Input: part model. Units: mm. Frame: model coordinates. A direction names the side the tool comes from. Coordinates: 2 decimals unless noted, no trailing zeros. Write each loop counter-clockwise with the first axis right and the second up, starting at its lowest first coordinate (ties: lowest second). Pieces come first, ordered by that corner, then holes.
1) Pin query (flat end, axial travel): pin 1 Ø5 at (y, z) = (6, -2.5) entering from -X; pin 2 Ø2 at (y, z) = (4, -4.5) entering from +X; pin 3 Ø3 at (x, y) = (17.89, 2.5) entering from -Z. Return the tip coordinate at first contact, or that it passes through.
2) Set-up query: faces 1 (the flat face through (16, 3, -18.625)), 2 (the cylindrical face through (19.63, 0.71, -20.9)), 3 (the flat face through (-2, 7, -5)). Return all of +Z, -Z, +X, -X, +Y, -Y with unobstructed straight access to the full face (end or side cutting, diameter ignored); none if empty.
3) Section query D-D (y = 5.5). Output: boundary loops of the cut face in (x, z).
4) Draft query along X for faces 4 (the cylindrical face through (0.158, 6.467, -2.465)), 5 (the cylindrical face through (-26.9, 4.25, -12.33)), 6 (the flat face through (-1, 10, -2)). Return one class per face: pulls with the +X half, pulls with the -X half, needs draft (parallel to the pull), parting line crosses it, or undercut.
5) Section query C-C (x = -6.5). Output: boundary loops of the cut face in (y, z), then the cut area to 3 significant figures.
6) Section query B-B (z = -20.75). State how many separate pieces and enclosed holes the cut face has, then the cut area to 3 significant figures.
7) Line query: L1, parallel to X at y = 2.5, z = -21.5; L2, parallel to Y at x = -19, z = -1.75; L3, parallel to Y at x = 18, z = -3. Output: solid intervals per line, ascending.
from build123d import *

# Parameters (mm, degrees)
BOSS_EXTRUDE1_DEPTH = 5
CUT_EXTRUDE1_REACH  = 39.584
SKETCH3_R           = 1.1
FILLET1_R           = 2.5
BOSS_EXTRUDE2_DEPTH = 5
SKETCH7_R           = 1.05
CUT_EXTRUDE3_DEPTH  = 5
FILLET2_R           = 5
CUT_EXTRUDE4_REACH  = 39.584
SKETCH8_W           = 5.5
SKETCH8_H           = 14.25
CHAMFER1_SIZE       = 5
FILLET3_R           = 3


with BuildPart() as part:
    # Sketch1 → Boss-Extrude1 (new body)
    with BuildSketch(Plane(origin=(0, 0, 0), x_dir=(1, 0, 0), z_dir=(0, 1, 0))):
        Polygon((-27.613970588, 0), (20.386029412, 0), (20.386029412, 23), (-27.613970588, 25), align=None)
    extrude(amount=BOSS_EXTRUDE1_DEPTH)

    # Cut-Extrude1: up to this plane
    cut_extrude1_end = Plane(origin=(-27.613970588, 5, -25), z_dir=(-0.04163054471218136, 0, 0.999133073092352))
    # Sketch3 → Cut-Extrude1 (cut, up to the surface)
    with BuildSketch(Plane.XY, mode=Mode.PRIVATE) as cut_extrude1_sk1:
        with Locations((-25.113970588, 2.5)):
            Circle(SKETCH3_R)
    cut_extrude1_tool1 = split(extrude(cut_extrude1_sk1.sketch, amount=-CUT_EXTRUDE1_REACH, mode=Mode.PRIVATE), bisect_by=cut_extrude1_end, keep=Keep.BOTH, mode=Mode.PRIVATE)
    add(cut_extrude1_tool1.solids().sort_by_distance((-25.113971, 2.5, 0))[0], mode=Mode.SUBTRACT)
    # Sketch3 → Cut-Extrude1 (cut, up to the surface)
    with BuildSketch(Plane.XY, mode=Mode.PRIVATE) as cut_extrude1_sk2:
        with Locations((17.886029412, 2.5)):
            Circle(SKETCH3_R)
    cut_extrude1_tool2 = split(extrude(cut_extrude1_sk2.sketch, amount=-CUT_EXTRUDE1_REACH, mode=Mode.PRIVATE), bisect_by=cut_extrude1_end, keep=Keep.BOTH, mode=Mode.PRIVATE)
    add(cut_extrude1_tool2.solids().sort_by_distance((17.886029, 2.5, 0))[0], mode=Mode.SUBTRACT)

    # Fillet1
    fillet1_edges = [part.edges().sort_by_distance(p)[0] for p in [
        (20.386029412, 0, -11.5),
        (20.386029412, 5, -11.5),
        (-27.613970588, 0, -12.5),
        (-27.613970588, 5, -12.5),
    ]]
    fillet(fillet1_edges, radius=FILLET1_R - 0.0001)  # a hair under: the kernel refuses the full size

    # Sketch4 → Boss-Extrude2 (add)
    with BuildSketch(Plane.XY):
        Polygon((-7.7850384, 5), (-2.7850384, 10), (2.886029412, 10), (2.886029412, 5), (-0.713970588, 5), (-4.249504494, 1.464466094), align=None)
    extrude(amount=-BOSS_EXTRUDE2_DEPTH)

    # Sketch7 → Cut-Extrude3 (cut)
    with BuildSketch(Plane.XY):
        with Locations((0.386029412, 7.492375144)):
            Circle(SKETCH7_R)
    extrude(amount=-CUT_EXTRUDE3_DEPTH, mode=Mode.SUBTRACT)

    # Fillet2
    fillet2_edges = [part.edges().sort_by_distance(p)[0] for p in [
        (2.886029412, 5, -2.5),
    ]]
    fillet(fillet2_edges, radius=FILLET2_R - 0.0001)  # a hair under: the kernel refuses the full size

    # Cut-Extrude4: up to this face of the body (flat: up to its plane)
    cut_extrude4_end = Plane(part.part.faces().sort_by_distance((-3.881478864, 0, -12.005573089))[0])
    # Sketch8 → Cut-Extrude4 (cut, up to the picked face)
    with BuildSketch(Plane(origin=(0, 5, 0), x_dir=(1, 0, 0), z_dir=(0, 1, 0)), mode=Mode.PRIVATE) as cut_extrude4_sk1:
        with Locations((17.636029412, 11.5)):
            Rectangle(SKETCH8_W, SKETCH8_H)
    cut_extrude4_tool1 = split(extrude(cut_extrude4_sk1.sketch, amount=-CUT_EXTRUDE4_REACH, mode=Mode.PRIVATE), bisect_by=cut_extrude4_end, keep=Keep.BOTH, mode=Mode.PRIVATE)
    add(cut_extrude4_tool1.solids().sort_by(Axis((17.636029, 5, -11.5), (0, -1, 0)))[0], mode=Mode.SUBTRACT)

    # Chamfer1
    chamfer1_edges = [part.edges().sort_by_distance(p)[0] for p in [
        (14.886029412, 5, -11.5),
    ]]
    chamfer(chamfer1_edges, length=CHAMFER1_SIZE - 0.0001)  # a hair under: the kernel refuses the full size

    # Fillet3
    fillet3_edges = [part.edges().sort_by_distance(p)[0] for p in [
        (2.886029412, 10, -2.5),
    ]]
    fillet(fillet3_edges, radius=FILLET3_R)


solid = part.part
Answer:
1. pin 1: stops at x = -27.41
1. pin 2: stops at x = 20.33
1. pin 3: stops at z = -23.17
2. face 1: +X, +Y
2. face 2: +Z, -Z, +X, -Y
2. face 3: -Z, +X, -X, +Y
3. outline: (-7.29, -5) - (5.71, -5) - (5.71, 0) - (-7.29, 0) - close
4. face 4: undercut
4. face 5: pulls with the -X half
4. face 6: needs draft
5. outline: (0, -24.12) - (5, -24.12) - (5, -5) - (6.29, -5) - (6.29, 0) - (0, 0) - close
5. area: 127 mm2
6. separate pieces: 1
6. enclosed holes: 2
6. area: 227 mm2
7. L1: x = -27.61 to -26.21, -24.01 to 16.79, 18.99 to 20.39
7. L2: y = 0 to 5
7. L3: y = 0 to 1.41, 3.59 to 5
